```python
from build123d import *

# Parameters (mm, degrees)
SKETCH2_W = 2.921
SKETCH2_H = 3.81
FILLET1_R = 1.651
FILLET3_R = 0.762


with BuildPart() as part:
    # Sketch2 → Revolve1 (revolve)
    with BuildSketch(Plane.XY):
        with Locations((36.6395, 1.905)):
            Rectangle(SKETCH2_W, SKETCH2_H)
    revolve(axis=Axis((0, -55, 0), (0, 1, 0)))

    # Fillet1
    fillet1_edges = [part.edges().sort_by_distance(p)[0] for p in [
        (-35.179, 3.81, 0),
        (-35.179, 0, 0),
    ]]
    fillet(fillet1_edges, radius=FILLET1_R)

    # Fillet3
    fillet3_edges = [part.edges().sort_by_distance(p)[0] for p in [
        (-38.1, 3.81, 0),
        (-38.1, 0, 0),
    ]]
    fillet(fillet3_edges, radius=FILLET3_R)


solid = part.part
```
Part model, mm, in its own coordinate system. Round coordinates to 2 decimals unless told otherwise and drop trailing zeros. Order: outer loops, then holes, each group sorted by start corner. A loop starts at its lowest first (then second) coordinate and runs counter-clockwise, first axis right, second up. Notation, with made-up numbers: M 41.5,70.25 L 93.5,70.25 A23 ccw 93.5,101.25 Z; hole C 62,-20.5 d9. An arc over 180 degrees is marked long. Put each result on its own line as item: value. Start each with the question number.
1. Drill centre lines: probe 1 along X at (y, z) = (1.95, 0); probe 2 along X at (y, z) = (1.05, -10.5). Where is each one in solid material? Low to high. Write a range as [from, to].
2. Slice it at B-B on z = 0. List the corners of the cut face in (x, y), then the cut area to 3 significant figures.
3. Drop a flat-ended pin along its axis: pin 1 (2 mm diameter, centred on y = 1.5, z = 29.5, fed in from +X). Give the stop position or say it passes through.
4. Two-plate mould, pull along X, no slides. Class faces 1 (the face through (-35.145, 1.909, -1.547)), 2 (the face through (-30.235, 1.921, 23.183)), 3 (the face through (-33, 0, -17)): +X half, -X half, draft (parallel to the pull), parting line (faces both ways), or undercut.
5. Slice it at A-A on x = 0. List the corners of the cut face in (y, z), then the cut area to 3 significant figures.
Findings:
1. probe 1: [-38.1, -35.18], [35.18, 38.1]
1. probe 2: [-36.62, -33.69], [33.69, 36.62]
2. outline: M -38.1,0.76 A0.76 ccw -37.34,0 L -36.83,0 A1.65 ccw -35.18,1.65 L -35.18,2.16 A1.65 ccw -36.83,3.81 L -37.34,3.81 A0.76 ccw -38.1,3.05 Z; M 35.18,1.65 A1.65 ccw 36.83,0 L 37.34,0 A0.76 ccw 38.1,0.76 L 38.1,3.05 A0.76 ccw 37.34,3.81 L 36.83,3.81 A1.65 ccw 35.18,2.16 Z
2. area: 19.4 mm2
3. pin 1: x = 25.29
4. face 1: undercut
4. face 2: parting line
4. face 3: draft
5. outline: M 0,-37.34 A0.76 ccw 0.76,-38.1 L 3.05,-38.1 A0.76 ccw 3.81,-37.34 L 3.81,-36.83 A1.65 ccw 2.16,-35.18 L 1.65,-35.18 A1.65 ccw 0,-36.83 Z; M 0,36.83 A1.65 ccw 1.65,35.18 L 2.16,35.18 A1.65 ccw 3.81,36.83 L 3.81,37.34 A0.76 ccw 3.05,38.1 L 0.76,38.1 A0.76 ccw 0,37.34 Z
5. area: 19.4 mm2
